For this review, take the finished solid that the model builds, in its own axes (mm). A direction names the side the tool comes from. Coordinates: 2 decimals unless noted, no trailing zeros. Write each loop counter-clockwise with the first axis right and the second up, starting at its lowest first coordinate (ties: lowest second). Pieces come first, ordered by that corner, then holes. Notation, with made-up numbers: M -11.75,-3.5 L 28.25,-3.5 A6 cw 28.25,2.5 Z; hole C 63.25,65 d3. An arc over 180 degrees is marked long. One line per question, with ' | ' between items.
from build123d import *

# Parameters (mm, degrees)
F1_DEPTH = 3
F3_D     = 3.3
F5_DEPTH = 25


with BuildPart() as f1:
    # F0 (on Top) → F1 (new body)
    with BuildSketch(Plane.XY):
        with BuildLine():
            Line((10.5, 17.5), (-10.5, 17.5))
            ThreePointArc((-10.5, 17.5), (-12.62132, 16.62132), (-13.5, 14.5))
            Line((-13.5, 14.5), (-13.5, -14.5))
            ThreePointArc((-13.5, -14.5), (-12.62132, -16.62132), (-10.5, -17.5))
            Line((-10.5, -17.5), (10.5, -17.5))
            ThreePointArc((10.5, -17.5), (12.62132, -16.62132), (13.5, -14.5))
            Line((13.5, -14.5), (13.5, 14.5))
            ThreePointArc((13.5, 14.5), (12.62132, 16.62132), (10.5, 17.5))
        make_face()
    extrude(amount=F1_DEPTH)

    # F3 (through all)
    with Locations(Plane.XY.offset(3)):
        with Locations((-9, 0), (9, 0)):
            Hole(F3_D / 2)

    # F4 (on face) → F5 (cut)
    with BuildSketch(Plane.XY.offset(3)):
        Polygon((6, 12.5), (-6, 12.5), (-6, -12.5), (-2.25, -12.5), (-2.25, -14.5), (2.25, -14.5), (2.25, -12.5), (6, -12.5), align=None)
    extrude(amount=-F5_DEPTH, mode=Mode.SUBTRACT)


solid = f1.part
1. Clearance check with a flat-ended pin moving along its axis: P1, Ø3, axis at x = 9, y = 0, coming from the -Z side. State where the tip first meets the part, or that it passes through.
Computed values:
P1: passes through
2. Take a section at B-B on x = -9. State the section outline as (y, z) points, plus the area to 3 significant figures.
Computed values:
outline: M -17.5,0 L -1.65,0 L -1.65,3 L -17.5,3 Z; M 1.65,0 L 17.5,0 L 17.5,3 L 1.65,3 Z | area: 95.1 mm2
3. Take a section at A-A on y = 0. State the section outline as (x, z) points, plus the area to 3 significant figures.
Computed values:
outline: M -13.5,0 L -10.65,0 L -10.65,3 L -13.5,3 Z; M -7.35,0 L -6,0 L -6,3 L -7.35,3 Z; M 6,0 L 7.35,0 L 7.35,3 L 6,3 Z; M 10.65,0 L 13.5,0 L 13.5,3 L 10.65,3 Z | area: 25.2 mm2
4. Take a section at C-C on z = 0.7. State the section outline as (x, y) points.
Computed values:
outline: M -13.5,-14.5 A3 ccw -10.5,-17.5 L 10.5,-17.5 A3 ccw 13.5,-14.5 L 13.5,14.5 A3 ccw 10.5,17.5 L -10.5,17.5 A3 ccw -13.5,14.5 Z; hole C -9,0 d3.3; hole M -6,-12.5 L -2.25,-12.5 L -2.25,-14.5 L 2.25,-14.5 L 2.25,-12.5 L 6,-12.5 L 6,12.5 L -6,12.5 Z; hole C 9,0 d3.3
5. Draft analysis for pull direction X (two halves, no side actions). For faces 3 (the flat face through (0, -17.5, 1)), 4 (the flat face through (6, 0, 2)), 5 (the cylindrical face through (12.64, 16.6, 1.48)), state which applies: pulls with the +X half, pulls with the -X half, needs draft (parallel to the pull), parting line crosses it, or undercut.
Computed values:
face 3: needs draft | face 4: undercut | face 5: pulls with the +X half
6. Machinability: for faces 1 (the cylindrical face through (12.6, -16.64, 1.48)), 2 (the flat face through (0, -14.5, 2)), which of the approach directions +Z, -Z, +X, -X, +Y, -Y give a long, thin tool a straight path to every point of the face, cutting with its end or side? Answer none if there is none.
Computed values:
face 1: +Z, -Z, +X, -Y | face 2: +Z, -Z
7. For line 1 along X through (y, z) = (-5, 1.75); line 2 along Y through (x, z) = (9, 0.8); line 3 along Y through (x, z) = (2, 0.4), list the stretches that pass through material, from the lowest coordinate up.
Computed values:
line 1: x = -13.5 to -6, 6 to 13.5 | line 2: y = -17.5 to -1.65, 1.65 to 17.5 | line 3: y = -17.5 to -14.5, 12.5 to 17.5
8. Take a section at D-D on x = -3. State the section outline as (y, z) points.
Computed values:
outline: M -17.5,0 L -12.5,0 L -12.5,3 L -17.5,3 Z; M 12.5,0 L 17.5,0 L 17.5,3 L 12.5,3 Z
